Autodesk Inventor part; units mm, degrees
ref_plane "YZ Plane" through (0, 0, 0) normal (1, 0, 0) x (0, 1, 0)
ref_plane "XZ Plane" through (0, 0, 0) normal (0, 1, 0) x (-1, 0, 0)
ref_plane "XY Plane" through (0, 0, 0) normal (0, 0, 1) x (1, 0, 0)
sketch "Эскиз1" plane through (0, 0, 0) normal (0, 0, 1) x (1, 0, 0)
  line L0 (-10, 0) -> (10, 0)
  line L1 (10, 0) -> (10, 14)
  line L2 (10, 14) -> (-10, 14)
  line L3 (-10, 14) -> (-10, 0)
  point P0 (0, 0)
  point P1 (0, 0)
  dimension "d0" = 20
  dimension "d1" = 14
extrude "Выдавливание1" add sketch "Эскиз1" along normal mid plane 79
sketch "Эскиз2" plane through (0, 0, 39.5) normal (0, 0, 1) x (1, 0, 0)
  circle A0 centre (6, 5) radius 1.4
  line L0 (-10, 0) -> (10, 0)
  line L1 (-10, 14) -> (-10, 0)
  point P0 (0, 0)
  point P1 (0, 0)
  dimension "d5" = 2.8
  dimension "d8" = 5
  dimension "d9" = 16
extrude "Выдавливание2" cut sketch "Эскиз2" against normal blind 14
sketch "Эскиз3" plane through (-10, 0, -39.5) normal (-1, 0, 0) x (0, 0, 1)
  circle A0 centre (71.5, 5) radius 1.4
  circle A1 centre (7.5, 5) radius 1.4
  line L0 (39.5, 0) -> (79, 0)
  line L1 (0, 14) -> (79, 14)
  line L2 (39.5, 0) -> (39.5, 14)
  dimension "d10" = 64
  dimension "d11" = 5
  dimension "d12" = 2.8
extrude "Выдавливание3" cut sketch "Эскиз3" against normal blind 16
mirror "Зеркальное отражение1" about plane through (0, 0, 0) normal (0, 0, 1) of "Выдавливание2"
sketch "Эскиз4" plane through (-10, 14, 39.5) normal (0, 1, 0) x (1, 0, 0)
  line L0 (0, 79) -> (0, 0)
  line L1 (0, 39.5) -> (20, 39.5)
  line L2 (20, 79) -> (20, 0)
  circle A0 centre (4, 64.5) radius 1.5
  circle A1 centre (4, 14.5) radius 1.5
  point P0 (10, 39.5)
  dimension "d15" = 50
  dimension "d16" = 3
  dimension "d17" = 4
extrude "Выдавливание4" cut sketch "Эскиз4" against normal through all
sketch "Эскиз5" plane through (-10, 0, 39.5) normal (-1, 0, 0) x (0, 0, 1)
  line L0 (-67.3, 10) -> (-61.7, 10)
  line L1 (-61.7, 10) -> (-61.7, 7.4)
  line L2 (-61.7, 7.4) -> (-67.3, 7.4)
  line L3 (-67.3, 7.4) -> (-67.3, 10)
  line L4 (-39.5, 0) -> (-39.5, 14)
  line L5 (-79, 14) -> (0, 14)
  line L6 (-11.7, 10) -> (-17.3, 10)
  line L7 (-17.3, 10) -> (-17.3, 7.4)
  line L8 (-17.3, 7.4) -> (-11.7, 7.4)
  line L9 (-11.7, 7.4) -> (-11.7, 10)
  line L10 (-63, 0) -> (-66, 0)
  line L11 (-66, 14) -> (-63, 14)
  point P0 (-64.5, 7.4)
  point P1 (-64.5, 0)
  dimension "d20" = 5.6
  dimension "d21" = 4
  dimension "d22" = 2.6
extrude "Выдавливание5" cut sketch "Эскиз5" against normal blind 7
properties part number "CupHolder"
Read the model definition and answer for the solid it produces. Units are mm, in the model's axes. A direction names the side the tool comes from. Give positions to 0.01 mm unless a question says otherwise; leave off trailing zeros. Order: outer loops, then holes, each group sorted by start corner. A loop starts at its lowest first (then second) coordinate and runs counter-clockwise, first axis right, second up. Notation, with made-up numbers: (-27, 29.25) -> (9, 29.25) arc R17 ccw to (9, 49.25) -> close; hole circle Ø10 at (65.5, -17.75). An arc over 180 degrees is marked (long way). One line per item, written item: value. Start each with the question number.
(1) The part is cut by section A-A (y = 5). Determine the outline of the cut face in (x, z).
(2) The part is cut by section C-C (y = 9.25). Determine the outline of the cut face in (x, z).
(3) The part is cut by section B-B (x = -6). State how many separate pieces and enclosed holes the cut face has, and give its area (3 significant figures).
(4) A tool of negligible diameter and unlimited length cuts with its end or side. For faces 4 (the flat face through (0, 0, -1)), 5 (the cylindrical face through (-6.195, 12.028, -26.487)), 6 (the flat face through (6, 5, 25.5)), 7 (the cylindrical face through (7.29, 5.54, -32.6)), 8 (the cylindrical face through (-2.11, 4.46, -30.71)), from which of +Z, -Z, +X, -X, +Y, -Y can it reach the whole face along a straight path? Write none if from no direction.
(5) Straight lines are drawn through the part: L1, parallel to Z at x = -6, y = 11.55; L2, parallel to Z at x = -4.5, y = 9.25; L3, parallel to X at y = 5, z = 34.25. For each, find the intervals that lie inside material, in ascending order.
(6) Flat-ended cylindrical pins translate along their axes: P1, Ø0.8, axis at x = 6.5, y = 5, coming from the -Z side; P2, Ø1.3, axis at y = 9, z = -26, coming from the -X side; P3, Ø3, axis at x = -5.5, z = -25.5, coming from the +Y side; P4, Ø1.8, axis at x = -6, z = 25, coming from the +Y side. Find the tip coordinate at first contact, or state that the pin passes through.
(7) For a pull along X with two mould halves and no side action, classify faces 1 (the flat face through (0, 7, -39.5)), 2 (the flat face through (-10, 7, -1)), 3 (the cylindrical face through (-6.195, 3.752, 23.513)) as released by +X, released by -X, zero draft, split by the parting line, or undercut.
(8) The part is cut by section D-D (z = -32). Determine the outline of the cut face in (x, y), and give its area (3 significant figures).
Taken from the geometry:
1. outline: (-10, -39.5) -> (4.6, -39.5) -> (4.6, -33.4) -> (-10, -33.4) -> close; (-10, -30.6) -> (4.6, -30.6) -> (4.6, -25.5) -> (7.4, -25.5) -> (7.4, -39.5) -> (10, -39.5) -> (10, 39.5) -> (7.4, 39.5) -> (7.4, 25.5) -> (4.6, 25.5) -> (4.6, 30.6) -> (-10, 30.6) -> close; (-10, 33.4) -> (4.6, 33.4) -> (4.6, 39.5) -> (-10, 39.5) -> close; hole circle Ø3 at (-6, -25); hole circle Ø3 at (-6, 25)
2. outline: (-10, -39.5) -> (10, -39.5) -> (10, 39.5) -> (-10, 39.5) -> (-10, 27.8) -> (-3, 27.8) -> (-3, 22.2) -> (-10, 22.2) -> (-10, -22.2) -> (-3, -22.2) -> (-3, -27.8) -> (-10, -27.8) -> close
3. separate pieces: 3
3. enclosed holes: 2
3. area: 996 mm^2
4. face 4: +Z, -Z, +X, -X, -Y
4. face 5: +Y, -Y
4. face 6: +Z
4. face 7: -Z
4. face 8: -X
5. L1: -39.5 to -26.5, -23.5 to 23.5, 26.5 to 39.5
5. L2: -39.5 to -27.8, -22.2 to 22.2, 27.8 to 39.5
5. L3: -10 to 4.6, 7.4 to 10
6. P1: z = -25.5
6. P2: x = -3
6. P3: y = 14
6. P4: through
7. face 1: zero draft
7. face 2: released by -X
7. face 3: undercut
8. outline: (-10, 0) -> (10, 0) -> (10, 14) -> (-10, 14) -> (-10, 6.4) -> (6, 6.4) arc R1.4 cw to (6, 3.6) -> (-10, 3.6) -> close
8. area: 232 mm^2
